CAD build for the part. Positions are in the model's coordinates, mm. Face numbers are marked on the shaded views. A direction names the side the tool comes from. Round coordinates to 2 decimals unless told otherwise and drop trailing zeros. Loops run counter-clockwise (first coordinate to the right, second up) from the corner with the lowest first, then second, coordinate; pieces in that order, holes last. Notation, with made-up numbers: M 44,71 L 82,71 A18 cw 82,106 Z; hole C 82.5,7.5 d6. An arc over 180 degrees is marked long. Use one line per item in the form item = value.
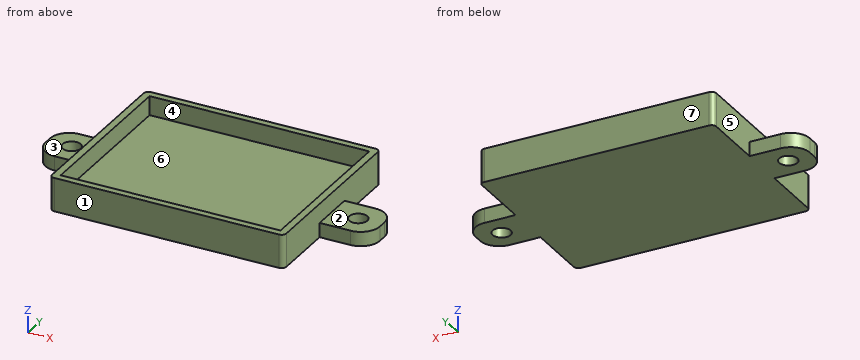
from build123d import *

# Parameters (mm, degrees)
BOX001_W          = 46
BOX001_H          = 35
BOX001_DEPTH      = 4
BOX_W             = 49
BOX_H             = 38
BOX_DEPTH         = 7
FILLET_R          = 1
CYLINDER001_R     = 1.9
CYLINDER001_DEPTH = 10
ARRAY002_X_COUNT  = 2
ARRAY002_X_PITCH  = 60
BOX005_W          = 70
BOX005_H          = 9.8
BOX005_DEPTH      = 3
FILLET002_R       = 4


with BuildPart() as internal_cube:
    # Box001 → Box001 (new body)
    with BuildSketch(Plane(origin=(1.5, 1.5, 3), x_dir=(1, 0, 0), z_dir=(0, 0, 1))):
        with Locations((23, 17.5)):
            Rectangle(BOX001_W, BOX001_H)
    extrude(amount=BOX001_DEPTH)


with BuildPart() as external_fillet:
    # Box → Box (new body)
    with BuildSketch(Plane.XY):
        with Locations((24.5, 19)):
            Rectangle(BOX_W, BOX_H)
    extrude(amount=BOX_DEPTH)

    # Fillet
    fillet_edges = [external_fillet.edges().sort_by_distance(p)[0] for p in [
        (0, 0, 3.5),
        (0, 38, 3.5),
        (49, 0, 3.5),
        (49, 38, 3.5),
    ]]
    fillet(fillet_edges, radius=FILLET_R)


with BuildPart() as attach_hole_array:
    # Cylinder001 → Cylinder001 (new body)
    with BuildSketch(Plane(origin=(5, 4.9, 0), x_dir=(1, 0, 0), z_dir=(0, 0, 1))):
        Circle(CYLINDER001_R)
    extrude(amount=CYLINDER001_DEPTH)

    # Array002 X: attach hole array ×2


with BuildPart() as attach_hole_array_1:
    add(attach_hole_array.part)
    with Locations(*[(i * ARRAY002_X_PITCH, 0, 0) for i in range(1, ARRAY002_X_COUNT)]):
        add(attach_hole_array.part)


with BuildPart() as bread_board_cut:
    # Box005 → Box005 (new body)
    with BuildSketch(Plane.XY):
        with Locations((35, 4.9)):
            Rectangle(BOX005_W, BOX005_H)
    extrude(amount=BOX005_DEPTH)

    # Fillet002
    fillet002_edges = [bread_board_cut.edges().sort_by_distance(p)[0] for p in [
        (0, 0, 1.5),
        (0, 9.8, 1.5),
        (70, 0, 1.5),
        (70, 9.8, 1.5),
    ]]
    fillet(fillet002_edges, radius=FILLET002_R)

    # Cut002: cut attach hole array
    add(attach_hole_array_1.part, mode=Mode.SUBTRACT)


with BuildPart() as bread_board_cut_1:
    # Cut002 placement: moved
    add(bread_board_cut.part.moved(Location((-10.5, 14.1, 0))))

    # Fusion: union external fillet
    add(external_fillet.part)

    # Cut: cut internal cube
    add(internal_cube.part, mode=Mode.SUBTRACT)


solid = bread_board_cut_1.part
1. Cut at B-B on y = 19. Write the cut outline in (x, z).
Completed:
outline = M -10.5,0 L -7.4,0 L -7.4,3 L -10.5,3 Z; M -3.6,0 L 52.6,0 L 52.6,3 L 49,3 L 49,7 L 47.5,7 L 47.5,3 L 1.5,3 L 1.5,7 L 0,7 L 0,3 L -3.6,3 Z; M 56.4,0 L 59.5,0 L 59.5,3 L 56.4,3 Z
2. Pull direction Y, two halves, no side cores. Call the marked faces 4, 5, 6 and 7: +Y half, -Y half, draft (parallel to the pull), parting line (faces both ways), or undercut.
Completed:
face_4 = undercut
face_5 = draft
face_6 = undercut
face_7 = +Y half
3. Cut at A-A on x = 54.5. Write the cut outline in (y, z).
Completed:
outline = M 14.1,0 L 17.1,0 L 17.1,3 L 14.1,3 Z; M 20.9,0 L 23.9,0 L 23.9,3 L 20.9,3 Z
4. Tool access for the marked faces 1, 2 and 3: list every direction of +Z, -Z, +X, -X, +Y, -Y with a clear straight run to the whole face (end or side of a thin tool).
Completed:
face_1 = +Z, -Z, +X, -X, -Y
face_2 = +Z, +X, +Y, -Y
face_3 = +Z, -X, +Y, -Y
5. Cut at D-D on y = 32. Write the cut outline in (x, z).
Completed:
outline = M 0,0 L 49,0 L 49,7 L 47.5,7 L 47.5,3 L 1.5,3 L 1.5,7 L 0,7 Z
6. Cut at C-C on z = 5.25. Write the cut outline in (x, y).
Completed:
outline = M 0,1 A1 ccw 1,0 L 48,0 A1 ccw 49,1 L 49,37 A1 ccw 48,38 L 1,38 A1 ccw 0,37 Z; hole M 1.5,1.5 L 47.5,1.5 L 47.5,36.5 L 1.5,36.5 Z
7. Drop flat-ended pins along their axis: P1, Ø1.2, axis at y = 22.5, z = 4.5, coming from the +X side; P2, Ø0.9, axis at x = -2, z = 1, coming from the +Y side; P3, Ø3, axis at x = -5.5, y = 19, coming from the +Z side; P4, Ø4, axis at y = 15.5, z = 3, coming from the -X side. Give the stop position or say it passes through.
Completed:
P1 = 49
P2 = 23.9
P3 = through
P4 = -10.45
8. Probe line 1 along X through (y, z) = (19, 1.8); line 2 along Y through (x, z) = (54.5, 1.75); line 3 along Y through (x, z) = (16, 4). List the from-to ranges inside material, lowest first. Write a range as from..to.
Completed:
line_1 = -10.5..-7.4, -3.6..52.6, 56.4..59.5
line_2 = 14.1..17.1, 20.9..23.9
line_3 = 0..1.5, 36.5..38
